Geometry: see drawing. Coordinates: mm, zero at the bounding-box minimum. A direction names the side the tool comes from. Give positions to 0.01 mm unless a question says otherwise; leave off trailing zeros. Write each loop counter-clockwise with the first axis right and the second up, starting at its lowest first coordinate (ties: lowest second). Pieces come first, ordered by that corner, then holes. Notation, with made-up numbers: (17.5, -4.75) - (35.5, -4.75) arc R17 ccw to (35.5, 17.25) - close; hole circle Ø9 at (63.25, 1). An arc over 180 degrees is marked (long way). One line per question, with ' | ' between items. Start each with the question number.
(1) Draft query along X for the marked faces 1, 2 and 3. Return one class per face: +X half, -X half, draft (parallel to the pull), parting line (faces both ways), or undercut.
(2) Ray query, line 1 (Y direction, x = 4, z = 5); line 2 (Y direction, x = 3.75, z = 2.5); line 3 (X direction, y = 9.25, z = 3.75) (1 decimal). Return the intervals inside material, ascending. Write a range as [from, to].
(3) Section D-D, the plane y = 8.75. Return loops of the section in (x, z) (1 decimal).
(4) Access query for the marked faces 4 and 5. Directions: +Z, -Z, +X, -X, +Y, -Y. A direction counts if a zero-diameter tool reaches every point of the face in a straight line with its end or side. Return the directions, or none.
(5) Section B-B, the plane z = 4.25. Return loops of the section in (x, y) (1 decimal).
(6) Section A-A, the plane y = 6.5. Return loops of the section in (x, z) (1 decimal).
(7) Section C-C, the plane x = 2.5. Return loops of the section in (y, z) (1 decimal).
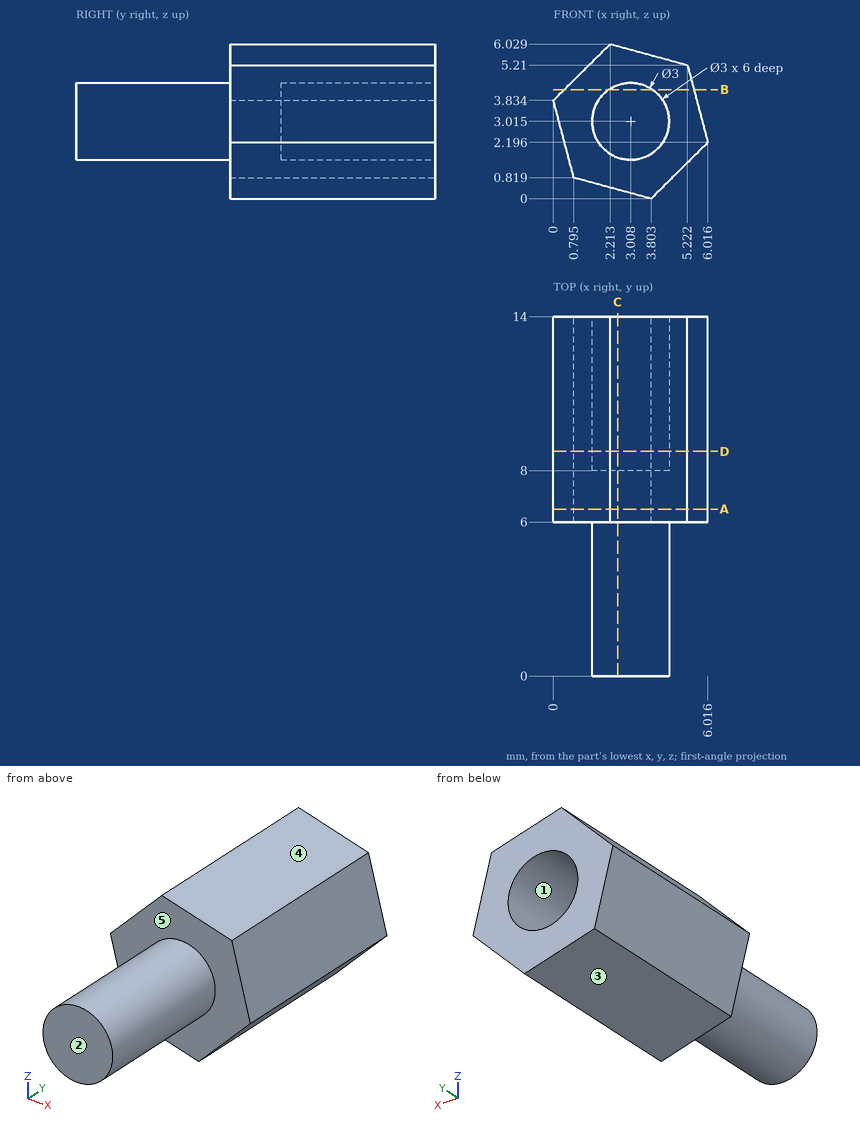
Check sheet entries:
1) face 1: undercut | face 2: draft | face 3: -X half
2) line 1: [6, 14] | line 2: [0, 8] | line 3: [0, 1.7], [4.3, 5.6]
3) outline: (0, 3.8) - (0.8, 0.8) - (3.8, 0) - (6, 2.2) - (5.2, 5.2) - (2.2, 6) - close; hole circle Ø3 at (3, 3)
4) face 4: +Z, +X, +Y, -Y | face 5: -Y
5) outline: (0.4, 6) - (2.2, 6) - (2.2, 0) - (3.9, 0) - (3.9, 6) - (5.5, 6) - (5.5, 14) - (3.9, 14) - (3.9, 8) - (2.2, 8) - (2.2, 14) - (0.4, 14) - close
6) outline: (0, 3.8) - (0.8, 0.8) - (3.8, 0) - (6, 2.2) - (5.2, 5.2) - (2.2, 6) - close
7) outline: (0, 1.6) - (6, 1.6) - (6, 0.4) - (14, 0.4) - (14, 1.6) - (8, 1.6) - (8, 4.4) - (14, 4.4) - (14, 6) - (6, 6) - (6, 4.4) - (0, 4.4) - close
